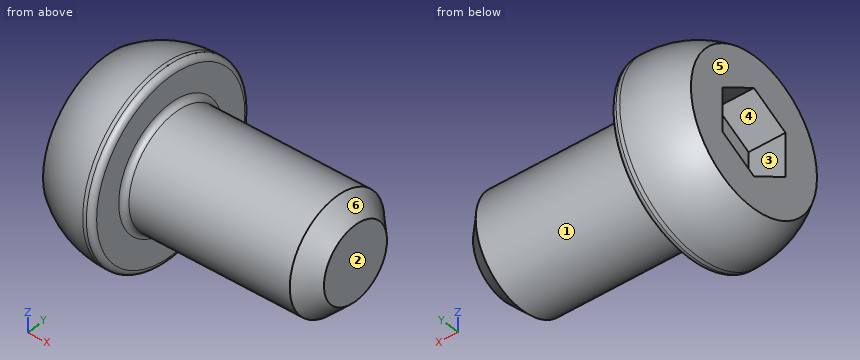
```python
from build123d import *

# Parameters (mm, degrees)
CUT_EXTRUDE_1_DEPTH = 2
FILLET_1_R          = 0.3
CHAMFER_1_SIZE      = 1


with BuildPart() as part:
    # Эскиз1 → Повернуть1 (revolve)
    with BuildSketch(Plane.XY):
        with BuildLine():
            Line((0, 0), (0, 4))
            ThreePointArc((0, 4), (1.41886117, 4.74341649), (3, 5))
            Line((3, 5), (3.5, 5))
            Line((3.5, 5), (3.5, 3))
            Line((3.5, 3), (13.5, 3))
            Line((13.5, 3), (13.5, 0))
            Line((13.5, 0), (0, 0))
        make_face()
    revolve(axis=Axis((13.5, 0, 0), (-1, 0, 0)))

    # Эскиз2 → Вырез-Вытянуть1 (cut)
    with BuildSketch(Plane.ZY):
        Polygon((1.154700538, 2), (-1.154700538, 2), (-2.309401077, 0), (-1.154700538, -2), (1.154700538, -2), (2.309401077, 0), align=None)
    extrude(amount=-CUT_EXTRUDE_1_DEPTH, mode=Mode.SUBTRACT)

    # Скругление1
    fillet_1_edges = [part.edges().sort_by_distance(p)[0] for p in [
        (3.5, -3, 0),
        (3.5, -5, 0),
    ]]
    fillet(fillet_1_edges, radius=FILLET_1_R)

    # Фаска1
    chamfer_1_edges = [part.edges().sort_by_distance(p)[0] for p in [
        (13.5, -3, 0),
    ]]
    chamfer(chamfer_1_edges, length=CHAMFER_1_SIZE)


solid = part.part
```
Geometry: final body of the model. Coordinates: model frame, mm. Face numbers are marked on the shaded views. A direction names the side the tool comes from. Coordinates: 2 decimals unless noted, no trailing zeros. Order: outer loops, then holes, each group sorted by start corner. A loop starts at its lowest first (then second) coordinate and runs counter-clockwise, first axis right, second up. Notation, with made-up numbers: (-15, -24) -> (1, -24) arc R20 ccw to (1, -13) -> close; hole circle Ø10 at (76.25, 21.25). An arc over 180 degrees is marked (long way). Answer in a Markdown table with one row per item.
Item 1: Contact query for flat-ended pins moving along their axis: P1, Ø1.5, axis at x = 5, z = 0.5, coming from the -Y side; P2, Ø2, axis at x = 3.5, y = 3, coming from the -Z side; P3, Ø1.6, axis at x = 0.5, z = 0, coming from the +Y side. Output: stop coordinate, or through.
Return value:
| item | result |
|---|---|
| P1 | stops at y = -3 |
| P2 | stops at z = -4.56 |
| P3 | stops at y = 4.7 |
Item 2: Section A-A on z = 0. Output: boundary loops of the cut face in (x, y), plus the area to 3 significant figures.
Return value:
| item | result |
|---|---|
| outline | (0, -4) arc R5 ccw to (3, -5) -> (3.2, -5) arc R0.3 ccw to (3.5, -4.7) -> (3.5, -3.3) arc R0.3 cw to (3.8, -3) -> (12.5, -3) -> (13.5, -2) -> (13.5, 2) -> (12.5, 3) -> (3.8, 3) arc R0.3 cw to (3.5, 3.3) -> (3.5, 4.7) arc R0.3 ccw to (3.2, 5) -> (3, 5) arc R5 ccw to (0, 4) -> (0, 2) -> (2, 2) -> (2, -2) -> (0, -2) -> close |
| area | 84.1 mm² |
Item 3: Access query for the marked faces 1, 2 and 3. Directions: +Z, -Z, +X, -X, +Y, -Y. A direction counts if a zero-diameter tool reaches every point of the face in a straight line with its end or side. Return the directions, or none.
Return value:
| item | result |
|---|---|
| face 1 | +X |
| face 2 | +Z, -Z, +X, +Y, -Y |
| face 3 | -X |
Item 4: Ray query, L1, parallel to X at y = 1, z = 0.25; L2, parallel to Y at x = 1, z = 0.75; L3, parallel to X at y = 3.5, z = -0.5. Return the intervals inside material, ascending.
Return value:
| item | result |
|---|---|
| L1 | x = 2 to 13.5 |
| L2 | y = -4.52 to -2, 2 to 4.52 |
| L3 | x = 0 to 3.5 |
Item 5: Draft query along Z for the marked faces 4, 5 and 6. Return one class per face: released by +Z, released by -Z, zero draft, split by the parting line, or undercut.
Return value:
| item | result |
|---|---|
| face 4 | undercut |
| face 5 | zero draft |
| face 6 | split by the parting line |
Item 6: Section B-B on x = 8.25. Output: boundary loops of the cut face in (y, z).
Return value:
| item | result |
|---|---|
| outline | circle Ø6 at (0, 0) |
